For this review, take the finished solid that the model builds, in its own axes (mm). Face numbers are marked on the shaded views. A direction names the side the tool comes from. Give positions to 0.01 mm unless a question says otherwise; leave off trailing zeros. Write each loop counter-clockwise with the first axis right and the second up, starting at its lowest first coordinate (ties: lowest second). Pieces come first, ordered by that corner, then holes. Notation, with made-up numbers: M -30.75,31.25 L 15.25,31.25 A24 ccw 15.25,49.25 Z; hole C 53,61.5 d10. An arc over 180 degrees is marked long. One line per item, written item: value. Start each with the question number.
Item 1: Clearance check with flat-ended pins moving along their axes: pin 1 Ø4 at (y, z) = (5, -6.5) entering from +X; pin 2 Ø2 at (x, y) = (-3, 2.5) entering from -Z; pin 3 Ø4.5 at (y, z) = (1, 1) entering from -X. State where each tip first meets the part, or that it passes through.
Item 2: To check wall thickness, follow probe 1 along Y at (x, z) = (-10, 0) (3 decimals); probe 2 along Y at (x, z) = (-14.65, 0); probe 3 along X at (y, z) = (13, 11.5) (3 decimals). State the ranges of each line that lie inside material, in increasing order.
Item 3: Consider section C-C, the plane x = -7. Write out the cut boundary in (y, z) (3 decimals).
Item 4: Tool access review of the marked faces 1 and 2: name each direction out of +Z, -Z, +X, -X, +Y, -Y from which nothing blocks a thin tool from reaching the whole face with its end or side.
Item 5: Consider section A-A, the plane y = 0. Give the number of separate pieces and of enclosed holes in the cut face, and give its area (3 significant figures).
Item 6: Mouldability with a two-part tool opening along Y and no side actions: class the marked faces 3, 4 and 5 as released by +Y, released by -Y, zero draft, split by the parting line, or undercut.
```python
from build123d import *

# Parameters (mm, degrees)
CUT_EXTRUDE1_DEPTH      = 32.270123521
CUT_EXTRUDE1_DEPTH_BACK = 32.270123521
SKETCH3_R               = 1.63195
SKETCH2_R               = 1.6
CUT_EXTRUDE2_DEPTH      = 32.270123571
CHAMFER1_SIZE           = 0.396875


with BuildPart() as part:
    # Sketch1 → Revolve1 (revolve)
    with BuildSketch(Plane.XY, mode=Mode.PRIVATE) as revolve1_sk:
        Polygon((0, 3.175), (0, 6.35), (-9.525, 6.35), (-9.525, 19.05), (-15.875, 19.05), (-15.875, 4.5), (-14.0716, 4.5), (-14.0716, 3.175), align=None)
    revolve(revolve1_sk.sketch.rotate(Axis((0, 0, 0), (-1, 0, 0)), 90), axis=Axis((0, 0, 0), (-1, 0, 0)))

    # Sketch3 → Cut-Extrude1 (cut, two sides: drawn at the far end of the back side and taken through both)
    with BuildSketch(Plane(origin=(0, 0, 0), x_dir=(1, 0, 0), z_dir=(0, 1, 0)).offset(-CUT_EXTRUDE1_DEPTH_BACK)):
        with Locations(Location((-4.7625, 0, 0), (0, 0, 270))):
            Circle(SKETCH3_R)
    extrude(amount=CUT_EXTRUDE1_DEPTH + CUT_EXTRUDE1_DEPTH_BACK, mode=Mode.SUBTRACT)

    # Sketch2 → Cut-Extrude2 (cut, through all)
    with BuildSketch(Plane.ZY.offset(15.875)):
        with Locations((-9.9568, 0)):
            Circle(SKETCH2_R)
        with Locations((0, 9.9568)):
            Circle(SKETCH2_R)
        with Locations((9.9568, 0)):
            Circle(SKETCH2_R)
        with Locations((0, -9.9568)):
            Circle(SKETCH2_R)
    extrude(amount=-CUT_EXTRUDE2_DEPTH, mode=Mode.SUBTRACT)

    # Chamfer1
    chamfer1_edges = [part.edges().sort_by_distance(p)[0] for p in [
        (0, 0, 6.35),
        (0, 0, 3.175),
        (-15.875, 0, 19.05),
        (-9.525, 0, 19.05),
    ]]
    chamfer(chamfer1_edges, length=CHAMFER1_SIZE)


solid = part.part
```
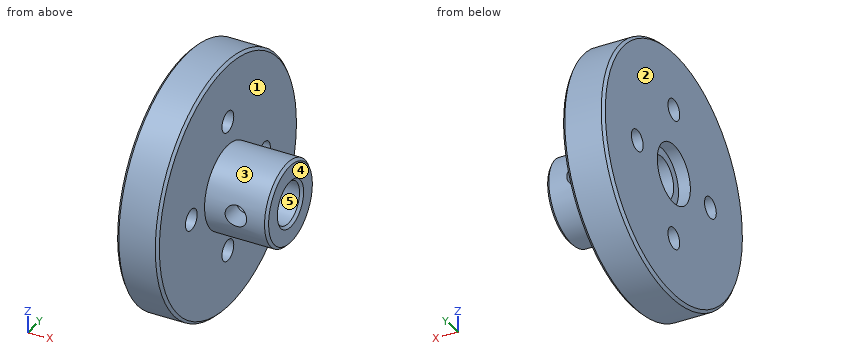
Model answer:
1. pin 1: stops at x = -0.25
1. pin 2: stops at z = -6.17
1. pin 3: stops at x = -14.07
2. probe 1: y = -19.05 to -11.557, -8.357 to -3.175, 3.175 to 8.357, 11.557 to 19.05
2. probe 2: y = -19.05 to -11.56, -8.36 to -4.5, 4.5 to 8.36, 11.56 to 19.05
2. probe 3: x = -15.875 to -9.525
3. outline: C 0,0 d12.7; hole C 0,0 d6.35
4. face 1: +X
4. face 2: +Z, -Z, -X, +Y, -Y
5. separate pieces: 4
5. enclosed holes: 0
5. area: 216 mm2
6. face 3: split by the parting line
6. face 4: zero draft
6. face 5: undercut
